Verification items for the finished model (mm, model axes). A direction names the side the tool comes from. Give positions to 0.01 mm unless a question says otherwise; leave off trailing zeros. Loops run counter-clockwise (first coordinate to the right, second up) from the corner with the lowest first, then second, coordinate; pieces in that order, holes last. Notation, with made-up numbers: M 71,72.5 L 124,72.5 A16 ccw 124,92.5 Z; hole C -31,2.5 d8. An arc over 180 degrees is marked long. Write each question's results on one line, items separated by ' | '. Start each with the question number.
```python
from build123d import *

# Parameters (mm, degrees)
SKETCH1_R           = 53
SKETCH1_R_2         = 51
BOSS_EXTRUDE2_DEPTH = 6
CUT_EXTRUDE1_DEPTH  = 10
CUT_EXTRUDE2_DEPTH  = 0.5


with BuildPart() as part:
    # Sketch1 → Boss-Extrude2 (new body)
    with BuildSketch(Plane(origin=(0, 0, 0), x_dir=(1, 0, 0), z_dir=(0, 1, 0))):
        with Locations(Location((0, 0, 0), (0, 0, 270))):
            Circle(SKETCH1_R)
        with Locations(Location((0, 0, 0), (0, 0, 270))):
            Circle(SKETCH1_R_2, mode=Mode.SUBTRACT)
    extrude(amount=BOSS_EXTRUDE2_DEPTH)

    # Sketch2 → Cut-Extrude1 (cut)
    with BuildSketch(Plane(origin=(0, 6, 0), x_dir=(1, 0, 0), z_dir=(0, 1, 0))):
        Polygon((0, 0), (0, 25.2), (76.826427625, 25.2), (76.826427625, -25.2), (0, -25.2), align=None)
    extrude(amount=-CUT_EXTRUDE1_DEPTH, mode=Mode.SUBTRACT)

    # Sketch3 → Cut-Extrude2 (cut)
    # profile 1 of 3: a face of its own
    with BuildSketch(Plane(origin=(0, 6, 0), x_dir=(1, 0, 0), z_dir=(0, 1, 0))):
        Polygon((-52.794871795, 1.695663061), (-52.794871795, 1.727564103), (-51.583333333, 1.727564103), (-51.583333333, 1.929487179), (-51.403846154, 1.929487179), (-51.403846154, 1.727564103), (-51, 1.727564103), (-51, 1.570512821), (-51.403846154, 1.570512821), (-51.403846154, 0.740384615), align=None)
        Polygon((-51.583333333, 1.570512821), (-52.343349359, 1.570512821), (-51.583333333, 1.048878205), align=None, mode=Mode.SUBTRACT)
    # profile 2 of 3: a face of its own
    with BuildSketch(Plane(origin=(0, 6, 0), x_dir=(1, 0, 0), z_dir=(0, 1, 0))):
        Polygon((-52.794871795, 0.349509215), (-52.794871795, 0.381410256), (-51.583333333, 0.381410256), (-51.583333333, 0.583333333), (-51.403846154, 0.583333333), (-51.403846154, 0.381410256), (-51, 0.381410256), (-51, 0.224358974), (-51.403846154, 0.224358974), (-51.403846154, -0.605769231), align=None)
        Polygon((-51.583333333, 0.224358974), (-52.343349359, 0.224358974), (-51.583333333, -0.297275641), align=None, mode=Mode.SUBTRACT)
    # profile 3 of 3: a face of its own
    with BuildSketch(Plane(origin=(0, 6, 0), x_dir=(1, 0, 0), z_dir=(0, 1, 0))):
        Polygon((-52.75, -1.579977965), (-52.75, -1.256410256), (-51, -1.256410256), (-51, -1.413461538), (-52.570512821, -1.413461538), (-52.570512821, -1.682692308), align=None)
    extrude(amount=-CUT_EXTRUDE2_DEPTH, mode=Mode.SUBTRACT)


solid = part.part
```
1. Depth check by flat-ended pin: pin 1 Ø0.7 at (x, y) = (45, 3) entering from +Z; pin 2 Ø3 at (y, z) = (5, 14) entering from -X; pin 3 Ø1 at (x, y) = (16.5, 5) entering from +Z. Enter the tip coordinate at first touch or a pass-through.
2. Release check for a two-part mould opening along Z. For faces 1 (the face through (-52.964, 2.958, -1.963)), 2 (the face through (-50.966, 2.958, -1.874)), 3 (the face through (-32, 0, -40)) record: released by +Z, released by -Z, zero draft, split by the parting line, or undercut.
3. Set-up check for faces 4 (the face through (45, 3, 25.2)), 5 (the face through (-32, 6, -40)): record each of +Z, -Z, +X, -X, +Y, -Y from which the full face is reachable in a straight line by a thin tool's end or side.
4. Section check D-D, the plane z = 20. Record the boundary of the cut face in (x, y), plus the area to 3 significant figures.
5. Section check A-A, the plane x = 0. Record the boundary of the cut face in (y, z), plus the area to 3 significant figures.
6. Section check C-C, the plane y = 2.7. Record the boundary of the cut face in (x, z).
7. Thickness scan on probe 1 along Z at (x, y) = (1, 5.6); probe 2 along X at (y, z) = (2.4, 39); probe 3 along Z at (x, y) = (-12, 0.6). Record the ranges inside material, lowest first.
8. Section check B-B, the plane z = -38. Record the boundary of the cut face in (x, y), plus the area to 3 significant figures.
Filled sheet:
1) pin 1: z = 28.55 | pin 2: x = -51.5 | pin 3: z = 50.53
2) face 1: split by the parting line | face 2: undercut | face 3: zero draft
3) face 4: +X, +Y, -Y | face 5: +Z, -Z, +X, -X, +Y
4) outline: M -49.08,0 L -46.91,0 L -46.91,6 L -49.08,6 Z | area: 13.0 mm2
5) outline: M 0,-53 L 6,-53 L 6,-51 L 0,-51 Z; M 0,51 L 6,51 L 6,53 L 0,53 Z | area: 24.0 mm2
6) outline: M 44.34,-25.2 A51 cw long 44.34,25.2 L 46.63,25.2 A53 ccw long 46.63,-25.2 Z
7) probe 1: -52.99 to -50.99, 50.99 to 52.99 | probe 2: -35.89 to -32.86, 32.86 to 35.89 | probe 3: -51.62 to -49.57, 49.57 to 51.62
8) outline: M -36.95,0 L -34.01,0 L -34.01,6 L -36.95,6 Z; M 34.01,0 L 36.95,0 L 36.95,6 L 34.01,6 Z | area: 35.2 mm2
